Can you work these out from the model? Positions are in its coordinate system, mm. Face numbers are marked on the shaded views. A direction names the side the tool comes from. Give positions to 0.01 mm unless a question says otherwise; leave off trailing zeros. Write each loop counter-clockwise with the first axis right and the second up, starting at its lowest first coordinate (ties: lowest second). Pieces come first, ordered by that corner, then holes.
from build123d import *

# Parameters (mm, degrees)
BOSS_EXTRUDE1_DEPTH = 14
SHELL1_T            = -2
BOSS_EXTRUDE2_DEPTH = 6.5
SKETCH3_R           = 4.19
CUT_EXTRUDE1_DEPTH  = 50.558046773
SKETCH8_R           = 3
SKETCH8_R_2         = 1.4
BOSS_EXTRUDE3_DEPTH = 3
SKETCH9_W           = 5
SKETCH9_H           = 4.5
BOSS_EXTRUDE4_DEPTH = 3
SKETCH10_R          = 3.5
CUT_EXTRUDE2_DEPTH  = 51.079936102


with BuildPart() as part:
    # Sketch1 → Boss-Extrude1 (new body)
    with BuildSketch(Plane.XY):
        Polygon((34, -14.083261121), (34, 14.083261121), (14.083261121, 34), (-14.083261121, 34), (-34, 14.083261121), (-34, -14.083261121), (-14.083261121, -34), (14.083261121, -34), align=None)
    extrude(amount=BOSS_EXTRUDE1_DEPTH)

    # Shell1
    shell1_openings = [part.faces().sort_by_distance(p)[0] for p in [
        (0, 0, 14),
    ]]
    offset(amount=SHELL1_T, openings=shell1_openings, kind=Kind.INTERSECTION)

    # Sketch2 → Boss-Extrude2 (add)
    with BuildSketch(Plane.XY.offset(2)):
        with BuildLine():
            Line((7, 32), (7, 25))
            ThreePointArc((7, 25), (0, 18), (-7, 25))
            Line((-7, 25), (-7, 32))
            Line((-7, 32), (-9, 32))
            Line((-9, 32), (-9, 25))
            ThreePointArc((-9, 25), (0, 16), (9, 25))
            Line((9, 25), (9, 32))
            Line((9, 32), (7, 32))
        make_face()
    extrude(amount=BOSS_EXTRUDE2_DEPTH)

    # Sketch3 → Cut-Extrude1 (cut, through all)
    with BuildSketch(Plane.XY.offset(2)):
        with Locations((0, 25)):
            Circle(SKETCH3_R)
    extrude(amount=-CUT_EXTRUDE1_DEPTH, mode=Mode.SUBTRACT)

    # Sketch8 → Boss-Extrude3 (add)
    with BuildSketch(Plane.XY.offset(2)):
        with Locations(Location((-5.2, -2, 0), (0, 0, 90))):
            Circle(SKETCH8_R)
        with Locations(Location((-5.2, -2, 0), (0, 0, 90))):
            Circle(SKETCH8_R_2, mode=Mode.SUBTRACT)
    boss_extrude3 = extrude(amount=BOSS_EXTRUDE3_DEPTH)

    # Mirror1: Boss-Extrude3 across plane
    add(boss_extrude3.mirror(Plane(origin=(0, 0, 0), x_dir=(0, 0, 1), z_dir=(1, 0, 0))))

    # Sketch6 → Cut-Revolve1 (revolve, cut)
    with BuildSketch(Plane(origin=(0, 0, 0), x_dir=(0, 0, -1), z_dir=(1, 0, 0)), mode=Mode.PRIVATE) as cut_revolve1_sk:
        Polygon((-6.3, 0.4), (0, 0.4), (0, -4.325), align=None)
    revolve(cut_revolve1_sk.sketch.rotate(Axis((0, 0.4, 6.3), (0, 0, -1)), 87.429020802), axis=Axis((0, 0.4, 6.3), (0, 0, -1)), mode=Mode.SUBTRACT)

    # Sketch9 → Boss-Extrude4 (add)
    with BuildSketch(Plane.XY.offset(2)):
        with Locations((-7.5, 9.25)):
            Rectangle(SKETCH9_W, SKETCH9_H)
        with Locations((7.5, 9.25)):
            Rectangle(SKETCH9_W, SKETCH9_H)
    extrude(amount=BOSS_EXTRUDE4_DEPTH)

    # Sketch10 → Cut-Extrude2 (cut, through all)
    with BuildSketch(Plane(origin=(0, 0, 0), x_dir=(-1, 0, 0), z_dir=(0, 0, -1))):
        with Locations((11.5, -9)):
            Circle(SKETCH10_R)
        with Locations((0, -11)):
            Circle(SKETCH10_R)
    extrude(amount=-CUT_EXTRUDE2_DEPTH, mode=Mode.SUBTRACT)


solid = part.part
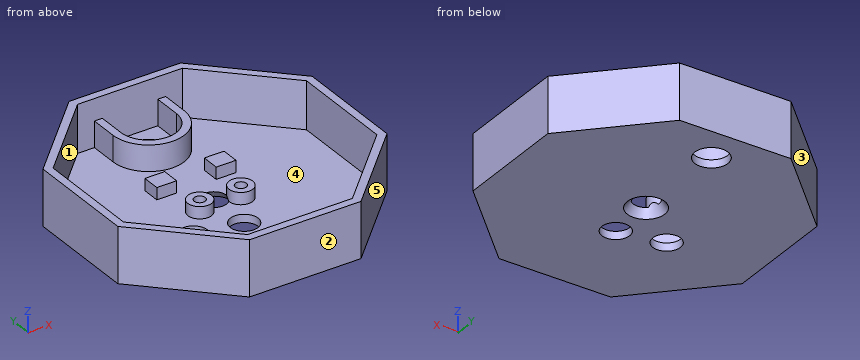
(1) Imagine slicing it at D-D, the plane x = 21.5. Write out the boundary of the cut face in (y, z).
Returned:
outline: (-26.58, 0) - (26.58, 0) - (26.58, 14) - (23.75, 14) - (23.75, 2) - (-23.75, 2) - (-23.75, 14) - (-26.58, 14) - close
(2) Imagine slicing it at B-B, the plane y = -11. Write out the boundary of the cut face in (x, z), plus the area to 3 significant figures.
Returned:
outline: (-34, 0) - (-14.37, 0) - (-14.37, 2) - (-32, 2) - (-32, 14) - (-34, 14) - close; (-8.63, 0) - (-3.5, 0) - (-3.5, 2) - (-8.63, 2) - close; (3.5, 0) - (34, 0) - (34, 14) - (32, 14) - (32, 2) - (3.5, 2) - close
area: 159 mm2
(3) Imagine slicing it at A-A, the plane x = -11.5. Write out the boundary of the cut face in (y, z), plus the area to 3 significant figures.
Returned:
outline: (-34, 0) - (-12.5, 0) - (-12.5, 2) - (-32, 2) - (-32, 14) - (-34, 14) - close; (-5.5, 0) - (34, 0) - (34, 14) - (32, 14) - (32, 2) - (-5.5, 2) - close
area: 170 mm2
(4) Will these pins go through, and if not, where does the flat tip stop? P1, Ø8, axis at x = -23.5, z = 9.5, coming from the -Y side; P2, Ø1.3, axis at x = 7, y = 8.5, coming from the +Z side; P3, Ø2, axis at x = -26, z = 6.5, coming from the -Y side; P4, Ø5.5, axis at x = 0, y = -11, coming from the +Z side.
Returned:
P1: stops at y = -28.58
P2: stops at z = 5
P3: stops at y = -23.08
P4: passes through
(5) If I drill on L1, parallel to X at y = -2, z = 3; L2, parallel to X at y = 7.5, z = 4.5; L3, parallel to Y at x = 9.5, z = 6.5, over which ranges is the centre line in solid material (lowest first)?
Returned:
L1: x = -34 to -32, -8.2 to -6.6, -3.8 to -2.2, 2.2 to 3.8, 6.6 to 8.2, 32 to 34
L2: x = -34 to -32, -10 to -5, 5 to 10, 32 to 34
L3: y = -34 to -32, 32 to 34
(6) For the marked faces 1 and 2, which set-ups out of +Z, -Z, +X, -X, +Y, -Y let a thin tool reach every point of the face, with its end or its side?
Returned:
face 1: +Z
face 2: +Z, -Z, +X, -X, -Y
(7) If we mould it in two halves opening along Y, with no side actions, what happens to the marked faces 3, 4 and 5? For each: +Y half, -Y half, draft (parallel to the pull), parting line (faces both ways), or undercut.
Returned:
face 3: +Y half
face 4: undercut
face 5: -Y half
(8) Imagine slicing it at C-C, the plane z = 10.75. Write out the boundary of the cut face in (x, y), plus the area to 3 significant figures.
Returned:
outline: (-34, -14.08) - (-14.08, -34) - (14.08, -34) - (34, -14.08) - (34, 14.08) - (14.08, 34) - (-14.08, 34) - (-34, 14.08) - close; hole (-32, -13.25) - (-13.25, -32) - (13.25, -32) - (32, -13.25) - (32, 13.25) - (13.25, 32) - (-13.25, 32) - (-32, 13.25) - close
area: 437 mm2
